Job drawing, mm, ordinate dimensions from the low corner. One solid piece. A direction names the side the tool comes from. Give positions to 0.01 mm unless a question says otherwise; leave off trailing zeros. Loops run counter-clockwise (first coordinate to the right, second up) from the corner with the lowest first, then second, coordinate; pieces in that order, holes last. Notation, with made-up numbers: (28.5, 66) - (58.5, 66) arc R19 cw to (58.5, 102) - close; hole circle Ø9 at (-6.5, 10). An arc over 180 degrees is marked (long way). Answer as CSV lines item,"result". Start each with the question number.
Item 1: Pin check, flat tips, straight feed: pin 1 (3.5 mm diameter, centred on x = 25, y = 30.5, fed in from -Z); pin 2 (5.5 mm diameter, centred on x = 140, y = 30.5, fed in from -Z). Stop position of each tip, or through.
Item 2: Saw through at D-D on y = 110. Give the cut face in (x, z).
Item 3: Tool access for the marked faces 4 and 5: list every direction of +Z, -Z, +X, -X, +Y, -Y with a clear straight run to the whole face (end or side of a thin tool).
Item 4: Drill centre lines: L1, parallel to Y at x = 22.4, z = 17.2; L2, parallel to X at y = 74, z = 15.85; L3, parallel to Y at x = 25, z = 17.05. Where is each one in solid material? Low to high. Write a range as from..to.
Item 5: Saw through at A-A on x = 82.5. Give the cut face in (y, z).
Item 6: Saw through at C-C on y = 56. Give the cut face in (x, z), plus the area to 3 significant figures.
Item 7: Pull direction X, two halves, no side cores. Call the marked faces 1, 2 and 3: pulls with the +X half, pulls with the -X half, needs draft (parallel to the pull), parting line crosses it, or undercut.
Item 8: Saw through at B-B on z = 11. Give the cut face in (x, y), plus the area to 3 significant figures.
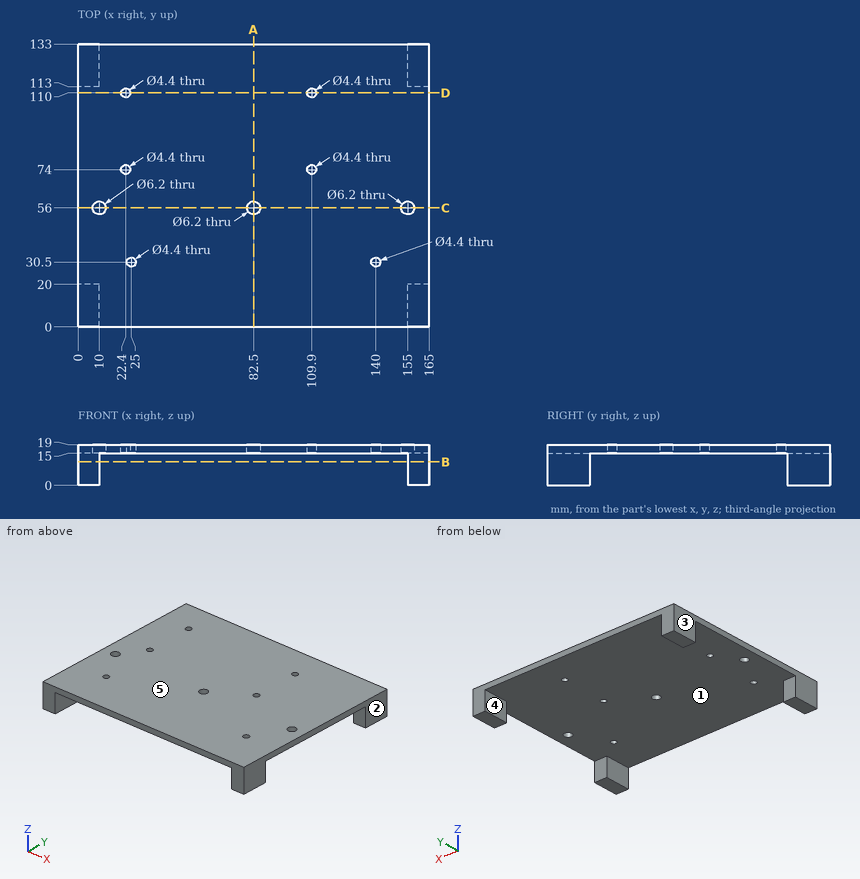
Responses:
1,pin 1,"through"
1,pin 2,"z = 15"
2,outline,"(0, 15) - (20.2, 15) - (20.2, 19) - (0, 19) - close; (24.6, 15) - (107.7, 15) - (107.7, 19) - (24.6, 19) - close; (112.1, 15) - (165, 15) - (165, 19) - (112.1, 19) - close"
3,face 4,"-Z, +Y, -Y"
3,face 5,"+Z, +X, -X, +Y, -Y"
4,L1,"0..71.8, 76.2..107.8, 112.2..133"
4,L2,"0..20.2, 24.6..107.7, 112.1..165"
4,L3,"0..28.3, 32.7..133"
5,outline,"(0, 15) - (52.9, 15) - (52.9, 19) - (0, 19) - close; (59.1, 15) - (133, 15) - (133, 19) - (59.1, 19) - close"
6,outline,"(0, 15) - (6.9, 15) - (6.9, 19) - (0, 19) - close; (13.1, 15) - (79.4, 15) - (79.4, 19) - (13.1, 19) - close; (85.6, 15) - (151.9, 15) - (151.9, 19) - (85.6, 19) - close; (158.1, 15) - (165, 15) - (165, 19) - (158.1, 19) - close"
6,area,"586 mm2"
7,face 1,"undercut"
7,face 2,"pulls with the +X half"
7,face 3,"pulls with the -X half"
8,outline,"(0, 0) - (10, 0) - (10, 20) - (0, 20) - close; (0, 113) - (10, 113) - (10, 133) - (0, 133) - close; (155, 0) - (165, 0) - (165, 20) - (155, 20) - close; (155, 113) - (165, 113) - (165, 133) - (155, 133) - close"
8,area,"800 mm2"
